```python
from build123d import *

# Parameters (mm, degrees)
BOSS_EXTRUDE1_DEPTH = 10
CHAMFER1_SIZE       = 0.5


with BuildPart() as part:
    # Sketch1 → Boss-Extrude1 (new body)
    with BuildSketch(Plane.XY):
        with BuildLine():
            Line((-9, 0), (-19, 0))
            ThreePointArc((-19, 0), (0, 19), (19, 0))
            Line((19, 0), (9, 0))
            ThreePointArc((9, 0), (0, 9), (-9, 0))
        make_face()
    extrude(amount=BOSS_EXTRUDE1_DEPTH)

    # Chamfer1
    chamfer1_edges = [part.edges().sort_by_distance(p)[0] for p in [
        (0, 19, 10),
        (0, 9, 10),
        (0, 19, 0),
        (0, 9, 0),
    ]]
    chamfer(chamfer1_edges, length=CHAMFER1_SIZE)


solid = part.part
```
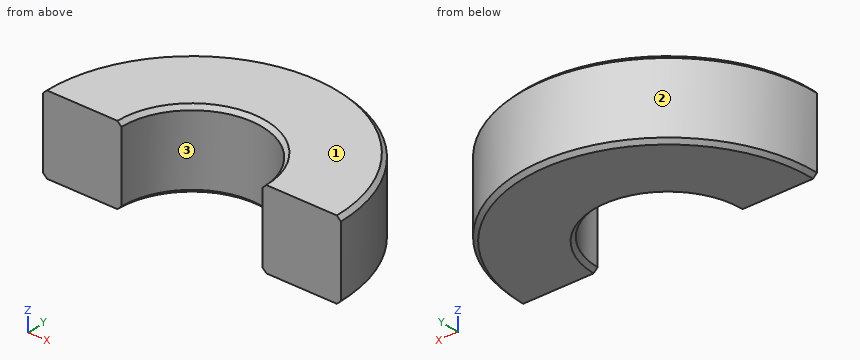
Geometry: final body of the model. Coordinates: model frame, mm. Face numbers are marked on the shaded views. Round coordinates to 2 decimals unless told otherwise and drop trailing zeros. Write each loop counter-clockwise with the first axis right and the second up, starting at its lowest first coordinate (ties: lowest second). Pieces come first, ordered by that corner, then holes. Notation, with made-up numbers: M 48,67 L 81,67 A4 ccw 81,74 Z; hole C 74,76 d8. An arc over 180 degrees is marked long. Answer in a Markdown table with one row per item. Add a question column.
(1) Contact query for flat-ended pins moving along their axis: pin 1 (2 mm diameter, centred on y = 13, z = 3.5, fed in from -X); pin 2 (4 mm diameter, centred on x = 5.5, y = 7.5, fed in from -Z); pin 3 (2 mm diameter, centred on x = 3.5, z = 4, fed in from +Y); pin 4 (5 mm diameter, centred on x = -1, y = 5, fed in from -Z). Output: stop coordinate, or through.
(2) Draft query along X for the marked faces 1, 2 and 3. Return one class per face: pulls with the +X half, pulls with the -X half, needs draft (parallel to the pull), parting line crosses it, or undercut.
(3) Cut plane A-A, the plane x = 0. Return the cut outline in (y, z), then the cut area to 3 significant figures.
(4) Cut plane B-B, the plane z = 3.5. Return the cut outline in (x, y).
(5) Ray query, L1, parallel to X at y = 6.25, z = 0.75; L2, parallel to Y at x = 0, z = 5.25; L3, parallel to Y at x = 1.5, z = 9. Return the intervals inside material, ascending.
Established:
| question | item | result |
|---|---|---|
| 1 | pin 1 | x = -14.73 |
| 1 | pin 2 | z = 0 |
| 1 | pin 3 | y = 18.83 |
| 1 | pin 4 | through |
| 2 | face 1 | needs draft |
| 2 | face 2 | parting line crosses it |
| 2 | face 3 | undercut |
| 3 | outline | M 9,0.5 L 9.5,0 L 18.5,0 L 19,0.5 L 19,9.5 L 18.5,10 L 9.5,10 L 9,9.5 Z |
| 3 | area | 99.5 mm² |
| 4 | outline | M -19,0 L -9,0 A9 cw 9,0 L 19,0 A19 ccw Z |
| 5 | L1 | -17.94 to -6.48, 6.48 to 17.94 |
| 5 | L2 | 9 to 19 |
| 5 | L3 | 8.87 to 18.94 |
